```python
from build123d import *

# Parameters (mm, degrees)
SALIENTE_EXTRUIR1_DEPTH  = 60
REDONDEO2_R              = 40
CROQUIS3_W               = 45
CROQUIS3_H               = 70
SALIENTE_EXTRUIR2_DEPTH  = 75
CROQUIS6_W               = 45
CROQUIS6_H               = 20
SALIENTE_EXTRUIR5_DEPTH  = 15
CROQUIS7_W               = 45
CROQUIS7_H               = 20
SALIENTE_EXTRUIR6_DEPTH  = 15
CROQUIS8_W               = 50
CROQUIS8_H               = 74
SALIENTE_EXTRUIR7_DEPTH  = 2.5
CROQUIS9_W               = 25
CROQUIS9_H               = 80
SALIENTE_EXTRUIR8_DEPTH  = 3
CROQUIS10_W              = 7
CROQUIS10_H              = 6
SALIENTE_EXTRUIR9_DEPTH  = 10
CROQUIS12_W              = 3
CROQUIS12_H              = 2
SALIENTE_EXTRUIR10_DEPTH = 25
MATRIZL1_COUNT           = 2
MATRIZL1_PITCH           = 65
CROQUIS13_R              = 10
SALIENTE_EXTRUIR11_DEPTH = 25
ESCALA3_SCALE            = 2.5


with BuildPart() as part:
    # Croquis2 → Saliente-Extruir1 (new body)
    with BuildSketch(Plane(origin=(0, 0, 0), x_dir=(1, 0, 0), z_dir=(0, 1, 0))):
        with BuildLine():
            Line((130, -45), (-130, -45))
            ThreePointArc((-130, -45), (-175, 0), (-130, 45))
            Line((-130, 45), (130, 45))
            Line((130, 45), (130, -45))
        make_face()
    extrude(amount=SALIENTE_EXTRUIR1_DEPTH)

    # Redondeo2
    redondeo2_edges = [part.edges().sort_by_distance(p)[0] for p in [
        (0, 0, -45),
        (0, 0, 45),
        (-175, 0, 0),
    ]]
    fillet(redondeo2_edges, radius=REDONDEO2_R)

    # Croquis3 → Saliente-Extruir2 (add)
    with BuildSketch(Plane(origin=(0, 60, 0), x_dir=(1, 0, 0), z_dir=(0, 1, 0))):
        with Locations((107.5, 0)):
            Rectangle(CROQUIS3_W, CROQUIS3_H)
    extrude(amount=SALIENTE_EXTRUIR2_DEPTH)

    # Croquis6 → Saliente-Extruir5 (add)
    with BuildSketch(Plane(origin=(0, 0, -35), x_dir=(-1, 0, 0), z_dir=(0, 0, -1))):
        with Locations((-107.5, 125)):
            Rectangle(CROQUIS6_W, CROQUIS6_H)
    extrude(amount=SALIENTE_EXTRUIR5_DEPTH)

    # Croquis7 → Saliente-Extruir6 (add)
    with BuildSketch(Plane.XY.offset(35)):
        with Locations((107.5, 125)):
            Rectangle(CROQUIS7_W, CROQUIS7_H)
    extrude(amount=SALIENTE_EXTRUIR6_DEPTH)

    # Croquis8 → Saliente-Extruir7 (add)
    with BuildSketch(Plane(origin=(0, 60, 0), x_dir=(1, 0, 0), z_dir=(0, 1, 0))):
        Rectangle(CROQUIS8_W, CROQUIS8_H)
        with Locations((-60, 0)):
            Rectangle(CROQUIS8_W, CROQUIS8_H)
        with Locations((60, 0)):
            Rectangle(CROQUIS8_W, CROQUIS8_H)
    extrude(amount=SALIENTE_EXTRUIR7_DEPTH)

    # Croquis9 → Saliente-Extruir8 (add)
    with BuildSketch(Plane(origin=(0, 135, 0), x_dir=(1, 0, 0), z_dir=(0, 1, 0))):
        with Locations((107.5, 0)):
            Rectangle(CROQUIS9_W, CROQUIS9_H)
    extrude(amount=SALIENTE_EXTRUIR8_DEPTH)

    # Croquis10 → Saliente-Extruir9 (add)
    with BuildSketch(Plane(origin=(0, 138, 0), x_dir=(1, 0, 0), z_dir=(0, 1, 0))):
        with Locations((107.5, -33)):
            Rectangle(CROQUIS10_W, CROQUIS10_H)
    saliente_extruir9 = extrude(amount=SALIENTE_EXTRUIR9_DEPTH)

    # Croquis12 → Saliente-Extruir10 (add)
    with BuildSketch(Plane(origin=(0, 148, 0), x_dir=(1, 0, 0), z_dir=(0, 1, 0))):
        with Locations((107.5, -33)):
            Rectangle(CROQUIS12_W, CROQUIS12_H)
    saliente_extruir10 = extrude(amount=SALIENTE_EXTRUIR10_DEPTH)

    # MatrizL1: Saliente-Extruir9, Saliente-Extruir10 ×2
    with Locations(*[(0, 0, -i * MATRIZL1_PITCH) for i in range(1, MATRIZL1_COUNT)]):
        add(saliente_extruir9)
        add(saliente_extruir10)

    # Croquis13 → Saliente-Extruir11 (add)
    with BuildSketch(Plane(origin=(0, 138, 0), x_dir=(1, 0, 0), z_dir=(0, 1, 0))):
        with Locations(Location((107.5, 0, 0), (0, 0, 270))):
            Circle(CROQUIS13_R)
    extrude(amount=SALIENTE_EXTRUIR11_DEPTH)


with BuildPart() as part_1:
    # Escala3: scaled about (4.422531692, 45.233244439, 0.000338602)
    add(part.part.scale(ESCALA3_SCALE).moved(Location((-6.633797538, -67.849866659, -0.000507903))))


solid = part_1.part
```
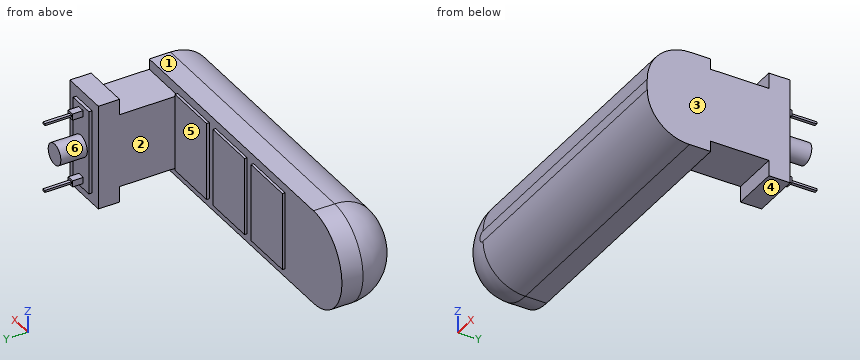
Geometry check sheet. Reference: the model listing, model coordinates, mm. Face numbers are marked on the shaded views. A direction names the side the tool comes from. Give positions to 0.01 mm unless a question says otherwise; leave off trailing zeros. Order: outer loops, then holes, each group sorted by start corner. A loop starts at its lowest first (then second) coordinate and runs counter-clockwise, first axis right, second up. Notation, with made-up numbers: (4.5, 27.5) - (9.5, 27.5) arc R5 cw to (9.5, 31.5) - close; hole circle Ø7 at (81.5, 50.25). An arc over 180 degrees is marked (long way). Write item = value, one per line. Start each with the question number.
1) Access from +Z, -Z, +X, -X, +Y, -Y to the whole of each face (thin tool, end or side, straight path). Record for the marked faces 1, 2 and 3.
2) Section check C-C (y = 41). Enter the section's corners in (x, z), then the cut area to 3 significant figures.
3) Section check A-A (x = -26.5). Enter the section's corners in (y, z).
4) Section check B-B (y = 324). Enter the section's corners in (x, z), then the cut area to 3 significant figures.
5) Scan lines: L1, parallel to X at y = 90, z = 12; L2, parallel to Z at x = -98.5, y = 87.5; L3, parallel to Z at x = 260, y = 33.5. Record each from-to range of solid material in increasing order.
6) Draft check along Z on the marked faces 4, 5 and 6. Enter one of: released by +Z, released by -Z, zero draft, split by the parting line, or undercut.
7) Gauge pin test, flat ends, axial feed: pin 1 Ø16.5 at (y, z) = (284.5, 84.5) entering from +X; pin 2 Ø2 at (x, y) = (277, 272.5) entering from -Z; pin 3 Ø14 at (x, y) = (259, 294.5) entering from -Z. Record the tip position at first contact, or that the pin passes through.
8) Section check D-D (x = -313). Enter the section's corners in (y, z), then the cut area to 3 significant figures.
Geometry check:
q1.face_1 = +Z, +X, -X, -Y
q1.face_2 = +Z, -Z, -X, +Y
q1.face_3 = +Z, -Z, +X, +Y, -Y
q2.outline = (-331.63, -112.5) - (318.37, -112.5) - (318.37, 112.5) - (-331.63, 112.5) arc R112.5 ccw to start
q2.area = 166,000 mm2
q3.outline = (-67.85, -12.5) arc R100 ccw to (32.15, -112.5) - (82.15, -112.5) - (82.15, -92.5) - (88.4, -92.5) - (88.4, 92.5) - (82.15, 92.5) - (82.15, 112.5) - (32.15, 112.5) arc R100 ccw to (-67.85, 12.5) - close
q4.outline = circle Ø50 at (262.12, 0); (258.37, -82.5) - (265.87, -82.5) - (265.87, -77.5) - (258.37, -77.5) - close; (258.37, 80) - (265.87, 80) - (265.87, 85) - (258.37, 85) - close
q4.area = 2,040 mm2
q5.L1 = 205.87 to 318.37
q5.L2 = -92.5 to 92.5
q5.L3 = -112.5 to 112.5
q6.face_4 = released by -Z
q6.face_5 = zero draft
q6.face_6 = undercut
q7.pin_1 = 293.37
q7.pin_2 = -100
q7.pin_3 = -87.5
q8.outline = (-67.85, -12.5) arc R100 ccw to (32.15, -112.5) - (82.15, -112.5) - (82.15, 112.5) - (32.15, 112.5) arc R100 ccw to (-67.85, 12.5) - close
q8.area = 29,500 mm2
